CAD build for the part. Positions are in the model's coordinates, mm. A direction names the side the tool comes from. Give positions to 0.01 mm unless a question says otherwise; leave off trailing zeros. Order: outer loops, then holes, each group sorted by start corner. A loop starts at its lowest first (then second) coordinate and runs counter-clockwise, first axis right, second up.
Item 1: Flat gauge pins, fed straight in: P1, Ø2, axis at x = 47.5, z = 35, coming from the -Y side; P2, Ø5.5, axis at x = 120.89, z = 45, coming from the +Y side; P3, Ø1.5, axis at x = 31.5, z = 6.5, coming from the +Y side; P4, Ø5, axis at x = 103.5, z = 22, coming from the -Y side. Where does each tip first touch, or does it go through?
Item 2: Band-saw the part on C-C on y = -347. Give the cut face in (x, z), plus the area to 3 significant figures.
Item 3: Band-saw the part on A-A on z = 45. Give the cut face in (x, y).
Item 4: Band-saw the part on B-B on x = 78. Give the cut face in (y, z), plus the area to 3 significant figures.
Item 5: Two-plate mould, pull along X, no slides. Class faces 1 (the flat face through (135.886, 70, 30)), 2 (the flat face through (23.26, 43.22, 29.58)), 3 (the cylindrical face through (95.38, 70.6, 15.2)): released by +X, released by -X, zero draft, split by the parting line, or undercut.
Item 6: Which spindle directions (+Z, -Z, +X, -X, +Y, -Y) get a long thin tool onto all of the face, cutting with end or side? Do faces 4 (the flat face through (10, -222, 30)), 5 (the cylindrical face through (94.457, 70.602, 42.262)). Say none if no direction does.
Item 7: Wall check: L1, parallel to X at y = -323.5, z = 23.5; L2, parallel to Y at x = 101.5, z = 10; L3, parallel to X at y = 53, z = 12. Give the ranges that are in metal, low to high.
```python
from build123d import *

# Parameters (mm, degrees)
BOSS_EXTRUDE1_DEPTH = 60
CUT_EXTRUDE1_REACH  = 543.312
SKETCH2_R           = 4.5


with BuildPart() as part:
    # Sketch1 → Boss-Extrude1 (new body)
    with BuildSketch(Plane.XY):
        Polygon((0, 0), (0, -445), (10, -445), (10, 0), (10, 6.847012111), (51.091785414, 65.532163543), (135.886114908, 65.532163543), (135.886114908, 75.532163543), (45.886114908, 75.532163543), (0, 10), align=None)
    extrude(amount=BOSS_EXTRUDE1_DEPTH)

    # Sketch2 → Cut-Extrude1 (cut, up to next)
    with BuildSketch(Plane(origin=(0, 75.532163543, 0), x_dir=(1, 0, 0), z_dir=(0, 1, 0)), mode=Mode.PRIVATE) as cut_extrude1_sk1:
        with Locations(Location((120.886114908, -15, 0), (0, 0, 180))):
            Circle(SKETCH2_R)
    cut_extrude1_tool1 = extrude(cut_extrude1_sk1.sketch, amount=-CUT_EXTRUDE1_REACH, mode=Mode.PRIVATE) & part.part
    # Sketch2 → Cut-Extrude1 (cut, up to next)
    with BuildSketch(Plane(origin=(0, 75.532163543, 0), x_dir=(1, 0, 0), z_dir=(0, 1, 0)), mode=Mode.PRIVATE) as cut_extrude1_sk2:
        with Locations(Location((120.886114908, -45, 0), (0, 0, 180))):
            Circle(SKETCH2_R)
    cut_extrude1_tool2 = extrude(cut_extrude1_sk2.sketch, amount=-CUT_EXTRUDE1_REACH, mode=Mode.PRIVATE) & part.part
    # Sketch2 → Cut-Extrude1 (cut, up to next)
    with BuildSketch(Plane(origin=(0, 75.532163543, 0), x_dir=(1, 0, 0), z_dir=(0, 1, 0)), mode=Mode.PRIVATE) as cut_extrude1_sk3:
        with Locations(Location((90.886114908, -15, 0), (0, 0, 180))):
            Circle(SKETCH2_R)
    cut_extrude1_tool3 = extrude(cut_extrude1_sk3.sketch, amount=-CUT_EXTRUDE1_REACH, mode=Mode.PRIVATE) & part.part
    # Sketch2 → Cut-Extrude1 (cut, up to next)
    with BuildSketch(Plane(origin=(0, 75.532163543, 0), x_dir=(1, 0, 0), z_dir=(0, 1, 0)), mode=Mode.PRIVATE) as cut_extrude1_sk4:
        with Locations(Location((90.886114908, -45, 0), (0, 0, 180))):
            Circle(SKETCH2_R)
    cut_extrude1_tool4 = extrude(cut_extrude1_sk4.sketch, amount=-CUT_EXTRUDE1_REACH, mode=Mode.PRIVATE) & part.part
    add(cut_extrude1_tool1.solids().sort_by_distance((120.886115, 75.532164, 15))[0], mode=Mode.SUBTRACT)
    add(cut_extrude1_tool2.solids().sort_by_distance((120.886115, 75.532164, 45))[0], mode=Mode.SUBTRACT)
    add(cut_extrude1_tool3.solids().sort_by_distance((90.886115, 75.532164, 15))[0], mode=Mode.SUBTRACT)
    add(cut_extrude1_tool4.solids().sort_by_distance((90.886115, 75.532164, 45))[0], mode=Mode.SUBTRACT)


solid = part.part
```
The answers:
1. P1: stops at y = 58.97
1. P2: passes through
1. P3: stops at y = 56.06
1. P4: stops at y = 65.53
2. outline: (0, 0) - (10, 0) - (10, 60) - (0, 60) - close
2. area: 600 mm2
3. outline: (0, -445) - (10, -445) - (10, 6.85) - (51.09, 65.53) - (86.39, 65.53) - (86.39, 75.53) - (45.89, 75.53) - (0, 10) - close; (95.39, 65.53) - (116.39, 65.53) - (116.39, 75.53) - (95.39, 75.53) - close; (125.39, 65.53) - (135.89, 65.53) - (135.89, 75.53) - (125.39, 75.53) - close
4. outline: (65.53, 0) - (75.53, 0) - (75.53, 60) - (65.53, 60) - close
4. area: 600 mm2
5. face 1: released by +X
5. face 2: released by -X
5. face 3: undercut
6. face 4: +Z, -Z, +X, -Y
6. face 5: +Y, -Y
7. L1: x = 0 to 10
7. L2: y = 65.53 to 75.53
7. L3: x = 30.11 to 42.32
